Design review of the part built by this model. Coordinates are the model's own, in mm. A direction names the side the tool comes from. Coordinates: 2 decimals unless noted, no trailing zeros. Order: outer loops, then holes, each group sorted by start corner. A loop starts at its lowest first (then second) coordinate and runs counter-clockwise, first axis right, second up.
from build123d import *

# Parameters (mm, degrees)
SKETCH1_W                    = 190
SKETCH1_H                    = 200
BASE_FLANGE1_DEPTH           = 5
EDGE_FLANGE1_STRIP_W         = 20.4
EDGE_FLANGE1_STRIP_H         = 5
EDGE_FLANGE1_STRIP_CUT_DEPTH = 190
EDGE_FLANGE1_DEPTH           = 190
EDGE_FLANGE2_STRIP_W         = 20.4
EDGE_FLANGE2_STRIP_H         = 5
EDGE_FLANGE2_STRIP_CUT_DEPTH = 190
EDGE_FLANGE2_DEPTH           = 190
CUT_EXTRUDE1_DEPTH           = 144.614066163
CUT_EXTRUDE1_DEPTH_BACK      = 144.614066163
SKETCH12_R                   = 35
CUT_EXTRUDE2_DEPTH           = 144.614066163
CUT_EXTRUDE2_DEPTH_BACK      = 144.614066163
SKETCH13_R                   = 8
CUT_EXTRUDE3_DEPTH           = 226
CUT_EXTRUDE3_DEPTH_BACK      = 226
SKETCH14_R                   = 7


# Sheet-metal steps are written as plain solids
with BuildPart() as part:
    # Sketch1 → Base-Flange1 (new body)
    with BuildSketch(Plane.XY):
        Rectangle(SKETCH1_W, SKETCH1_H)
    extrude(amount=-BASE_FLANGE1_DEPTH)

    # Edge-Flange1 strip (across the edge) → Edge-Flange1 strip cut (cut)
    with BuildSketch(Plane(origin=(-95, 100, -5), x_dir=(0, -1, 0), z_dir=(1, 0, 0))):
        with Locations((-5, -2.5)):
            Rectangle(EDGE_FLANGE1_STRIP_W, EDGE_FLANGE1_STRIP_H)
    extrude(amount=EDGE_FLANGE1_STRIP_CUT_DEPTH, mode=Mode.SUBTRACT)

    # Edge-Flange1 section (across the edge) → Edge-Flange1 (add)
    with BuildSketch(Plane(origin=(-95, 100, -5), x_dir=(0, -1, 0), z_dir=(1, 0, 0))):
        with BuildLine():
            Line((0, 0.2), (0, 35))
            Line((0, 35), (5, 35))
            Line((5, 35), (5, 0.2))
            ThreePointArc((5, 0.2), (5.058578644, 0.058578644), (5.2, 0))
            Line((5.2, 0), (5.2, -5))
            ThreePointArc((5.2, -5), (1.523044738, -3.476955262), (0, 0.2))
        make_face()
    extrude(amount=EDGE_FLANGE1_DEPTH)

    # Edge-Flange2 strip (across the edge) → Edge-Flange2 strip cut (cut)
    with BuildSketch(Plane(origin=(95, -100, -5), x_dir=(0, 1, 0), z_dir=(-1, 0, 0))):
        with Locations((-5, -2.5)):
            Rectangle(EDGE_FLANGE2_STRIP_W, EDGE_FLANGE2_STRIP_H)
    extrude(amount=EDGE_FLANGE2_STRIP_CUT_DEPTH, mode=Mode.SUBTRACT)

    # Edge-Flange2 section (across the edge) → Edge-Flange2 (add)
    with BuildSketch(Plane(origin=(95, -100, -5), x_dir=(0, 1, 0), z_dir=(-1, 0, 0))):
        with BuildLine():
            Line((0, 0.2), (0, 35))
            Line((0, 35), (5, 35))
            Line((5, 35), (5, 0.2))
            ThreePointArc((5, 0.2), (5.058578644, 0.058578644), (5.2, 0))
            Line((5.2, 0), (5.2, -5))
            ThreePointArc((5.2, -5), (1.523044738, -3.476955262), (0, 0.2))
        make_face()
    extrude(amount=EDGE_FLANGE2_DEPTH)

    # Sketch12 → Cut-Extrude1 (cut, two sides: drawn at the far end of the back side and taken through both)
    with BuildSketch(Plane.XY.offset(-CUT_EXTRUDE1_DEPTH_BACK)):
        with Locations(Location((0, 0, 0), (0, 0, 180))):
            Circle(SKETCH12_R)
    extrude(amount=CUT_EXTRUDE1_DEPTH + CUT_EXTRUDE1_DEPTH_BACK, mode=Mode.SUBTRACT)

    # Sketch13 → Cut-Extrude2 (cut, two sides: drawn at the far end of the back side and taken through both)
    with BuildSketch(Plane.XY.offset(-CUT_EXTRUDE2_DEPTH_BACK)):
        with Locations(Location((55.5, 55.5, 0), (0, 0, 180))):
            Circle(SKETCH13_R)
        with Locations(Location((-55.5, 55.5, 0), (0, 0, 180))):
            Circle(SKETCH13_R)
        with Locations(Location((-55.5, -55.5, 0), (0, 0, 180))):
            Circle(SKETCH13_R)
        with Locations(Location((55.5, -55.5, 0), (0, 0, 180))):
            Circle(SKETCH13_R)
    extrude(amount=CUT_EXTRUDE2_DEPTH + CUT_EXTRUDE2_DEPTH_BACK, mode=Mode.SUBTRACT)

    # Sketch14 → Cut-Extrude3 (cut, two sides: drawn at the far end of the back side and taken through both)
    with BuildSketch(Plane(origin=(0, -100, 0), x_dir=(-1, 0, 0), z_dir=(0, -1, 0)).offset(-CUT_EXTRUDE3_DEPTH_BACK)):
        with Locations(Location((75, 25, 0), (0, 0, 270))):
            Circle(SKETCH14_R)
        with Locations(Location((-75, 25, 0), (0, 0, 270))):
            Circle(SKETCH14_R)
    extrude(amount=CUT_EXTRUDE3_DEPTH + CUT_EXTRUDE3_DEPTH_BACK, mode=Mode.SUBTRACT)


solid = part.part
1. To check wall thickness, follow line 1 (X direction, y = 55, z = -1); line 2 (X direction, y = 97.5, z = -25); line 3 (Y direction, x = -57.5, z = -17). State the ranges of each line that lie inside material, in increasing order.
2. Add section B-B (x = 75). Give the boundary of the cut face in (y, z), and give its area (3 significant figures).
3. Mouldability with a two-part tool opening along Y and no side actions: class faces 3 (the cylindrical face through (56.541, -63.432, -2.535)), 4 (the cylindrical face through (1.33, -98.436, -1.483)), 5 (the flat face through (-95, 0, -2)) as pulls with the +Y half, pulls with the -Y half, needs draft (parallel to the pull), parting line crosses it, or undercut.
4. Add section A-A (x = 0). Give the boundary of the cut face in (y, z), and give its area (3 significant figures).
5. Add section C-C (z = -25). Give the boundary of the cut face in (x, y).
6. Add section D-D (y = -13.5). Give the boundary of the cut face in (x, z), and give its area (3 significant figures).
7. Insertion check: pin 1 (14.5 mm diameter, centred on x = -55.5, y = 55.5, fed in from +Z); pin 2 (1.5 mm diameter, centred on x = 9.5, y = -55, fed in from -Z). Each pin has a flat end and moves straight along its axis. Give the tip position at first contact, or say it passes through.
8. For faces 1 (the flat face through (-1, 100, -22)), 2 (the flat face through (-1, -41, -5)), list the 3-axis set-ups (+Z, -Z, +X, -X, +Y, -Y) from which the entire face can be reached by the end or side of a thin tool; tool diameter is ignored.
Solution:
1. line 1: x = -95 to -63.48, -47.52 to 47.52, 63.48 to 95
1. line 2: x = -95 to -82, -68 to 68, 82 to 95
1. line 3: y = -100 to -95, 95 to 100
2. outline: (-100, -40) - (-95, -40) - (-95, -32) - (-100, -32) - close; (-100, -18) - (-95, -18) - (-95, -5.2) arc R0.2 cw to (-94.8, -5) - (94.8, -5) arc R0.2 cw to (95, -5.2) - (95, -18) - (100, -18) - (100, -5.2) arc R5.2 ccw to (94.8, 0) - (-94.8, 0) arc R5.2 ccw to (-100, -5.2) - close; (95, -40) - (100, -40) - (100, -32) - (95, -32) - close
2. area: 1,200 mm2
3. face 3: undercut
3. face 4: pulls with the -Y half
3. face 5: needs draft
4. outline: (-100, -40) - (-95, -40) - (-95, -5.2) arc R0.2 cw to (-94.8, -5) - (-35, -5) - (-35, 0) - (-94.8, 0) arc R5.2 ccw to (-100, -5.2) - close; (35, -5) - (94.8, -5) arc R0.2 cw to (95, -5.2) - (95, -40) - (100, -40) - (100, -5.2) arc R5.2 ccw to (94.8, 0) - (35, 0) - close
4. area: 988 mm2
5. outline: (-95, -100) - (-82, -100) - (-82, -95) - (-95, -95) - close; (-95, 95) - (-82, 95) - (-82, 100) - (-95, 100) - close; (-68, -100) - (68, -100) - (68, -95) - (-68, -95) - close; (-68, 95) - (68, 95) - (68, 100) - (-68, 100) - close; (82, -100) - (95, -100) - (95, -95) - (82, -95) - close; (82, 95) - (95, 95) - (95, 100) - (82, 100) - close
6. outline: (-95, -5) - (-32.29, -5) - (-32.29, 0) - (-95, 0) - close; (32.29, -5) - (95, -5) - (95, 0) - (32.29, 0) - close
6. area: 627 mm2
7. pin 1: passes through
7. pin 2: stops at z = -5
8. face 1: +Z, -Z, +X, -X, +Y
8. face 2: -Z, +X, -X
